CAD build for the part. Positions are in the model's coordinates, mm. Face numbers are marked on the shaded views. A direction names the side the tool comes from. Give positions to 0.01 mm unless a question says otherwise; leave off trailing zeros. Order: outer loops, then holes, each group sorted by start corner. A loop starts at its lowest first (then second) coordinate and runs counter-clockwise, first axis right, second up. Notation, with made-up numbers: (-11.5, 83) -> (21.5, 83) arc R35 ccw to (21.5, 117) -> close; hole circle Ø2 at (81, -11). An arc over 180 degrees is marked (long way). Answer as CSV lines item,"result".
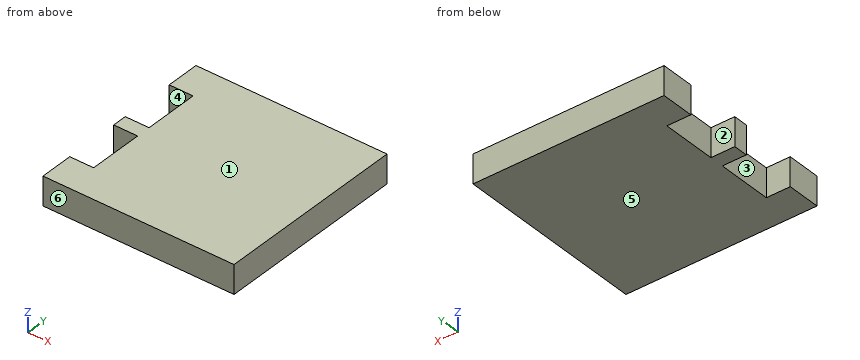
```python
from build123d import *

# Parameters (mm, degrees)
SKETCH1_W           = 45
SKETCH1_H           = 40
BOSS_EXTRUDE1_DEPTH = 6
SKETCH2_W           = 5
SKETCH2_H           = 11.5
CUT_EXTRUDE1_DEPTH  = 6
SKETCH3_W           = 5
SKETCH3_H           = 9
SKETCH3_H_2         = 3
CUT_EXTRUDE3_DEPTH  = 6
SKETCH4_W           = 8.469823435
SKETCH4_H           = 40.874478331
CUT_EXTRUDE4_DEPTH  = 6


with BuildPart() as part:
    # Sketch1 → Boss-Extrude1 (new body)
    with BuildSketch(Plane.XY):
        with Locations((-3.25562701, 9.807073955)):
            Rectangle(SKETCH1_W, SKETCH1_H)
    extrude(amount=BOSS_EXTRUDE1_DEPTH)

    # Sketch2 → Cut-Extrude1 (cut)
    with BuildSketch(Plane.XY.offset(6)):
        with Locations((-23.25562701, 17.057073955)):
            Rectangle(SKETCH2_W, SKETCH2_H)
        with Locations((-23.25562701, 2.557073955)):
            Rectangle(SKETCH2_W, SKETCH2_H)
    extrude(amount=-CUT_EXTRUDE1_DEPTH, mode=Mode.SUBTRACT)

    # Sketch3 → Cut-Extrude3 (cut)
    with BuildSketch(Plane.XY.offset(6)):
        with Locations((16.74437299, 25.307073955)):
            Rectangle(SKETCH3_W, SKETCH3_H)
        with Locations((16.74437299, 9.807073955)):
            Rectangle(SKETCH3_W, SKETCH3_H_2)
        with Locations((16.74437299, -5.692926045)):
            Rectangle(SKETCH3_W, SKETCH3_H)
    extrude(amount=-CUT_EXTRUDE3_DEPTH, mode=Mode.SUBTRACT)

    # Sketch4 → Cut-Extrude4 (cut)
    with BuildSketch(Plane.XY.offset(6)):
        with Locations((18.479284707, 9.36983479)):
            Rectangle(SKETCH4_W, SKETCH4_H)
    extrude(amount=-CUT_EXTRUDE4_DEPTH, mode=Mode.SUBTRACT)


solid = part.part
```
1) Which spindle directions (+Z, -Z, +X, -X, +Y, -Y) get a long thin tool onto all of the face, cutting with end or side? Do the marked faces 1 and 2. Say none if no direction does.
Data:
face 1,"+Z, +X, -X, +Y, -Y"
face 2,"+Z, -Z, -X"
2) Pull direction Y, two halves, no side cores. Call the marked faces 3, 4, 5 and 6: pulls with the +Y half, pulls with the -Y half, needs draft (parallel to the pull), parting line crosses it, or undercut.
Data:
face 3,"undercut"
face 4,"undercut"
face 5,"needs draft"
face 6,"pulls with the -Y half"
3) Band-saw the part on B-B, the plane y = 6.5. Write the cut outline in (x, z).
Data:
outline,"(-20.76, 0) -> (14.24, 0) -> (14.24, 6) -> (-20.76, 6) -> close"
4) Band-saw the part on A-A, the plane z = 0.8. Write the cut outline in (x, y).
Data:
outline,"(-25.76, -10.19) -> (14.24, -10.19) -> (14.24, 29.81) -> (-25.76, 29.81) -> (-25.76, 22.81) -> (-20.76, 22.81) -> (-20.76, 11.31) -> (-25.76, 11.31) -> (-25.76, 8.31) -> (-20.76, 8.31) -> (-20.76, -3.19) -> (-25.76, -3.19) -> close"
5) Wall check: line 1 along Y through (x, z) = (-22.5, 4.1); line 2 along X through (y, z) = (7.5, 3.5). Give the ranges that are in metal, low to high. Write a range as [from, to].
Data:
line 1,"y = [-10.19, -3.19], [8.31, 11.31], [22.81, 29.81]"
line 2,"x = [-20.76, 14.24]"
